Can you work these out from the model? Positions are in its coordinate system, mm. Face numbers are marked on the shaded views. A direction names the side the tool comes from. Round coordinates to 2 decimals unless told otherwise and drop trailing zeros. Order: outer loops, then holes, each group sorted by start corner. A loop starts at its lowest first (then second) coordinate and runs counter-clockwise, first axis right, second up.
Q1. Will these pins go through, and if not, where does the flat tip stop? P1, Ø2.5, axis at x = 10.61, z = -10.61, coming from the -Y side; P2, Ø2.5, axis at x = -10.61, z = -10.61, coming from the +Y side; P3, Ø7.5, axis at x = 0, z = 0, coming from the -Y side; P4, Ø3, axis at x = 11.5, y = 0.5, coming from the +Z side.
Q2. If we section it at B-B (z = 0): Please give me the cut outline in (x, y), plus the area to 3 significant figures.
Q3. If I drill on line 1 (X direction, y = 3.25, z = 9.5); line 2 (Z direction, x = 11.5, y = 2.75); line 3 (Y direction, x = -2, z = 16), over which ranges is the centre line in solid material (lowest first)?
Q4. We'd pull the mould along Z, two halves only. Please class the marked faces 4, 5 and 6: pulls with the +Z half, pulls with the -Z half, needs draft (parallel to the pull), parting line crosses it, or undercut.
Q5. If we section it at A-A (x = 0): Please give me the cut outline in (y, z), plus the area to 3 significant figures.
Q6. For the marked faces 1, 2 and 3, which set-ups out of +Z, -Z, +X, -X, +Y, -Y let a thin tool reach every point of the face, with its end or its side?
Q7. If we section it at C-C (y = 6.5): Please give me the cut outline in (x, z).
Q8. If we section it at D-D (z = 10): Please give me the cut outline in (x, y), plus the area to 3 significant figures.
from build123d import *

# Parameters (mm, degrees)
SKETCH1_R              = 18.5
BOSS_EXTRUDE1_DEPTH    = 6
SKETCH2_R              = 18.5
SKETCH2_R_2            = 17.5
BOSS_EXTRUDE2_DEPTH    = 1
M14X1_5_TAPPED_HOLE1_D = 12.5
SKETCH5_R              = 1.5
CUT_EXTRUDE1_DEPTH     = 4


with BuildPart() as part:
    # Sketch1 → Boss-Extrude1 (new body)
    with BuildSketch(Plane(origin=(0, 0, 0), x_dir=(1, 0, 0), z_dir=(0, 1, 0))):
        with Locations(Location((0, 0, 0), (0, 0, 270))):
            Circle(SKETCH1_R)
    extrude(amount=BOSS_EXTRUDE1_DEPTH)

    # Sketch2 → Boss-Extrude2 (add)
    with BuildSketch(Plane(origin=(0, 6, 0), x_dir=(1, 0, 0), z_dir=(0, 1, 0))):
        with Locations(Location((0, 0, 0), (0, 0, 270))):
            Circle(SKETCH2_R)
        with Locations(Location((0, 0, 0), (0, 0, 270))):
            Circle(SKETCH2_R_2, mode=Mode.SUBTRACT)
    extrude(amount=BOSS_EXTRUDE2_DEPTH)

    # M14x1.5 Tapped Hole1 (through all)
    with Locations(Plane(origin=(0, 6, 0), x_dir=(1, 0, 0), z_dir=(0, 1, 0))):
        with Locations((0, 0)):
            Hole(M14X1_5_TAPPED_HOLE1_D / 2)

    # Sketch5 → Cut-Extrude1 (cut)
    with BuildSketch(Plane.XZ):
        with Locations(Location((-10.606601718, 10.606601718, 0), (0, 0, 270))):
            Circle(SKETCH5_R)
        with Locations(Location((10.606601718, 10.606601718, 0), (0, 0, 270))):
            Circle(SKETCH5_R)
        with Locations(Location((10.606601718, -10.606601718, 0), (0, 0, 270))):
            Circle(SKETCH5_R)
        with Locations(Location((-10.606601718, -10.606601718, 0), (0, 0, 270))):
            Circle(SKETCH5_R)
    extrude(amount=-CUT_EXTRUDE1_DEPTH, mode=Mode.SUBTRACT)


solid = part.part
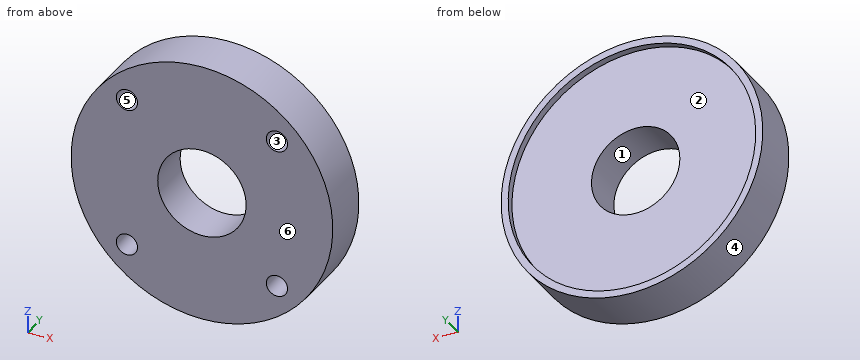
Solution:
1. P1: stops at y = 4
1. P2: stops at y = 6
1. P3: passes through
1. P4: stops at z = 15.56
2. outline: (-18.5, 0) - (-6.25, 0) - (-6.25, 6) - (-17.5, 6) - (-17.5, 7) - (-18.5, 7) - close; (6.25, 0) - (18.5, 0) - (18.5, 7) - (17.5, 7) - (17.5, 6) - (6.25, 6) - close
2. area: 149 mm2
3. line 1: x = -15.87 to -11.62, -9.59 to 9.59, 11.62 to 15.87
3. line 2: z = -14.49 to -11.81, -9.4 to 9.4, 11.81 to 14.49
3. line 3: y = 0 to 6
4. face 4: parting line crosses it
4. face 5: undercut
4. face 6: needs draft
5. outline: (0, -18.5) - (7, -18.5) - (7, -17.5) - (6, -17.5) - (6, -6.25) - (0, -6.25) - close; (0, 6.25) - (6, 6.25) - (6, 17.5) - (7, 17.5) - (7, 18.5) - (0, 18.5) - close
5. area: 149 mm2
6. face 1: +Y, -Y
6. face 2: +Y
6. face 3: -Y
7. outline: circle Ø37 at (0, 0); hole circle Ø35 at (0, 0)
8. outline: (-15.56, 0) - (-11.98, 0) - (-11.98, 4) - (-9.23, 4) - (-9.23, 0) - (9.23, 0) - (9.23, 4) - (11.98, 4) - (11.98, 0) - (15.56, 0) - (15.56, 7) - (14.36, 7) - (14.36, 6) - (-14.36, 6) - (-14.36, 7) - (-15.56, 7) - close
8. area: 167 mm2
